Build history of the part. All positions in model axes, mm. A direction names the side the tool comes from. Give positions to 0.01 mm unless a question says otherwise; leave off trailing zeros. Write each loop counter-clockwise with the first axis right and the second up, starting at its lowest first coordinate (ties: lowest second). Pieces come first, ordered by that corner, then holes.
from build123d import *

# Parameters (mm, degrees)
SKETCH_1_W          = 15
SKETCH_1_H          = 5.08
EXTRUDE_1_DEPTH     = 9
SKETCH_2_R          = 0.75
EXTRUDE_2_DEPTH     = 8.5
SKETCH_3_R          = 1.5
CUT_EXTRUDE_1_DEPTH = 2
EXTRUDE_3_DEPTH     = 0.75


with BuildPart() as part:
    # 草图1 → 凸台-拉伸1 (new body)
    with BuildSketch(Plane.XY):
        Rectangle(SKETCH_1_W, SKETCH_1_H)
    extrude(amount=EXTRUDE_1_DEPTH)

    # 草图2 → 凸台-拉伸2 (add)
    with BuildSketch(Plane.XY.offset(9)):
        with BuildLine():
            Line((6.5, -2.54), (6.5, -2.04))
            ThreePointArc((6.5, -2.04), (7.12789195, 0), (6.5, 2.04))
            Line((6.5, 2.04), (6.5, 2.54))
            Line((6.5, 2.54), (1, 2.54))
            Line((1, 2.54), (1, 1.25))
            Line((1, 1.25), (1.5, 1.25))
            Line((1.5, 1.25), (1.5, -1.25))
            Line((1.5, -1.25), (1, -1.25))
            Line((1, -1.25), (1, -2.54))
            Line((1, -2.54), (6.5, -2.54))
        make_face()
        with Locations((3.5, 0)):
            Circle(SKETCH_2_R, mode=Mode.SUBTRACT)
    extrude(amount=EXTRUDE_2_DEPTH)

    # 草图3 → 切除-拉伸1 (cut)
    with BuildSketch(Plane.XY.offset(17.5)):
        with Locations((3.5, 0)):
            Circle(SKETCH_3_R)
    extrude(amount=-CUT_EXTRUDE_1_DEPTH, mode=Mode.SUBTRACT)

    # 草图4 → 凸台-拉伸3 (add)
    with BuildSketch(Plane.XZ.offset(2.54)):
        Polygon((-4, 9), (-4, 8.307126737), (-1, 8.307126737), (-1, 9), (-1, 13), (-3, 13), align=None)
    extrude_3 = extrude(amount=-EXTRUDE_3_DEPTH)

    # 镜向1: 凸台-拉伸3 across plane
    add(extrude_3.mirror(Plane.ZX))


solid = part.part
1. Saw through at C-C on y = 0. Give the cut face in (x, z), plus the area to 3 significant figures.
2. Drill centre lines: line 1 along Y through (x, z) = (3.5, 12.5); line 2 along X through (y, z) = (0, 13.25); line 3 along Y through (x, z) = (-1.5, 11). Where is each one in solid material? Low to high.
3. Drop flat-ended pins along their axis: pin 1 (1.5 mm diameter, centred on x = -3.5, y = 1, fed in from +Z); pin 2 (2.5 mm diameter, centred on x = 3.5, y = 0, fed in from +Z); pin 3 (0.6 mm diameter, centred on x = -2, y = -2, fed in from +Z). Give the stop position or say it passes through.
4. Saw through at A-A on z = 16.5. Give the cut face in (x, y), plus the area to 3 significant figures.
5. Saw through at D-D on z = 13.25. Give the cut face in (x, y), plus the area to 3 significant figures.
6. Mould opens along X. For faces 1 (the face through (0, 0, 0)), 2 (the face through (-3.5, -2.2, 11)), 3 (the face through (1, -2, 13)), 4 (the face through (2.75, 0.03, 12.2)) say: pulls with the +X half, pulls with the -X half, needs draft (parallel to the pull), parting line crosses it, or undercut.
7. 3-axis set-ups, long thin cutter, end or side, ignore diameter. For faces 5 (the face through (-7.5, 0, 4)), 6 (the face through (7.3, 0, 9)), 7 (the face through (4.886, -0.575, 16.514)), 8 (the face through (-2, 1.79, 11)): which of +Z, -Z, +X, -X, +Y, -Y reach the whole face in a straight line?
8. Saw through at B-B on x = 3.5. Give the cut face in (y, z).
Outcome:
1. outline: (-7.5, 0) - (7.5, 0) - (7.5, 9) - (7.13, 9) - (7.13, 17.5) - (5, 17.5) - (5, 15.5) - (4.25, 15.5) - (4.25, 9) - (2.75, 9) - (2.75, 15.5) - (2, 15.5) - (2, 17.5) - (1.5, 17.5) - (1.5, 9) - (-7.5, 9) - close
1. area: 167 mm2
2. line 1: y = -2.54 to -0.75, 0.75 to 2.54
2. line 2: x = 1.5 to 2.75, 4.25 to 7.13
2. line 3: y = -2.54 to -1.79, 1.79 to 2.54
3. pin 1: stops at z = 9
3. pin 2: stops at z = 15.5
3. pin 3: stops at z = 13
4. outline: (1, -2.54) - (6.5, -2.54) - (6.5, -2.04) arc R3.63 ccw to (6.5, 2.04) - (6.5, 2.54) - (1, 2.54) - (1, 1.25) - (1.5, 1.25) - (1.5, -1.25) - (1, -1.25) - close; hole circle Ø3 at (3.5, 0)
4. area: 21.4 mm2
5. outline: (1, -2.54) - (6.5, -2.54) - (6.5, -2.04) arc R3.63 ccw to (6.5, 2.04) - (6.5, 2.54) - (1, 2.54) - (1, 1.25) - (1.5, 1.25) - (1.5, -1.25) - (1, -1.25) - close; hole circle Ø1.5 at (3.5, 0)
5. area: 26.7 mm2
6. face 1: needs draft
6. face 2: pulls with the -X half
6. face 3: undercut
6. face 4: undercut
7. face 5: +Z, -Z, -X, +Y, -Y
7. face 6: +Z, +X
7. face 7: +Z
7. face 8: +Z, -X
8. outline: (-2.54, 0) - (2.54, 0) - (2.54, 17.5) - (1.5, 17.5) - (1.5, 15.5) - (0.75, 15.5) - (0.75, 9) - (-0.75, 9) - (-0.75, 15.5) - (-1.5, 15.5) - (-1.5, 17.5) - (-2.54, 17.5) - close
